Part model, mm, in its own coordinate system. A direction names the side the tool comes from. Coordinates: 2 decimals unless noted, no trailing zeros. Loops run counter-clockwise (first coordinate to the right, second up) from the corner with the lowest first, then second, coordinate; pieces in that order, holes last. Notation, with made-up numbers: (-19, -32.75) -> (30, -32.75) arc R16 cw to (30, -4.75) -> close; hole circle Ø5 at (72, 36). An arc over 180 degrees is marked (long way). Use one line per item in the form item = value. Start each with the question number.
(1) 3-axis set-ups, long thin cutter, end or side, ignore diameter. For faces 4 (the flat face through (35.91, 2, 0.5)), 5 (the flat face through (10.3, -2.658, 0.5)), 6 (the flat face through (10.6, 5.542, 0.5)), 7 (the flat face through (-5.8, -7.658, 0.5)): which of +Z, -Z, +X, -X, +Y, -Y reach the whole face in a straight line?
(2) Band-saw the part on A-A on z = 0.55. Count the separate pieces of the cut face and the enclosed holes in it, then the cut area to 3 significant figures.
(3) Band-saw the part on B-B on y = 2. Give the cut face in (x, z), then the cut area to 3 significant figures.
(4) Mould opens along X. For faces 1 (the flat face through (37.2, 6.542, 0.5)), 2 (the flat face through (40.208, -0.7, 0.5)), 3 (the cylindrical face through (38.46, -0.03, 0.51)) say: +X half, -X half, draft (parallel to the pull), parting line (faces both ways), or undercut.
(5) Band-saw the part on C-C on x = -5. Give the cut face in (y, z), then the cut area to 3 significant figures.
(6) Pin check, flat tips, straight feed: P1, Ø0.5, axis at x = 7.5, z = 0.5, coming from the +Y side; P2, Ø0.5, axis at x = 10, z = 0.5, coming from the -Y side. Stop position of each tip, or through.
(7) Drill centre lines: L1, parallel to X at y = 2, z = 0.85; L2, parallel to X at y = -6, z = 0.4; L3, parallel to X at y = 0, z = 0.2. Where is each one in solid material? Low to high. Write a range as [from, to].
```python
from build123d import *

# Parameters (mm, degrees)
F0_W     = 3
F0_H     = 5
F1_DEPTH = 1
F2_R     = 1.49999
F3_R     = 1.5


# Not quite as in the source:
# - a fillet or chamfer is up to 0.001 mm smaller than in the source, because OpenCascade refuses the exact size


with BuildPart() as f1:
    # F0 (on Top) → F1 (new body)
    with BuildSketch(Plane.XY):
        Polygon((-13.5924067289, 6.5421499412), (-19.5924067289, 6.5421499412), (-19.5924067289, -7.6578500588), (8.3075932711, -7.6578500588), (8.3075932711, -2.6578500588), (12.3075932711, -2.6578500588), (12.3075932711, -7.6578500588), (40.2075932711, -7.6578500588), (40.2075932711, 6.5421499412), (34.2075932711, 6.5421499412), (34.2075932711, 5.5421499412), (-13.5924067289, 5.5421499412), align=None)
        with Locations((-16.332133919, 2.0421499412)):
            Rectangle(F0_W, F0_H, mode=Mode.SUBTRACT)
        with Locations((37.4102636576, 2.0421499412)):
            Rectangle(F0_W, F0_H, mode=Mode.SUBTRACT)
    extrude(amount=F1_DEPTH)

    # F2 (radius 1.5 in the source; OpenCascade refuses exactly that, so slightly less here)
    f2_edges = [f1.edges().sort_by_distance(p)[0] for p in [
        (-17.832134, 4.54215, 0.5),
        (-14.832134, 4.54215, 0.5),
        (-14.832134, -0.45785, 0.5),
        (-17.832134, -0.45785, 0.5),
        (38.910264, 4.54215, 0.5),
        (35.910264, 4.54215, 0.5),
        (35.910264, -0.45785, 0.5),
        (38.910264, -0.45785, 0.5),
    ]]
    fillet(f2_edges, radius=F2_R)

    # F3
    f3_edges = [f1.edges().sort_by_distance(p)[0] for p in [
        (8.307593, -2.65785, 0.5),
        (12.307593, -2.65785, 0.5),
    ]]
    fillet(f3_edges, radius=F3_R)


solid = f1.part
```
A:
q1.face_4 = +Z, -Z
q1.face_5 = +Z, -Z, -Y
q1.face_6 = +Z, -Z, +Y
q1.face_7 = +Z, -Z, +X, -X, -Y
q2.separate_pieces = 1
q2.enclosed_holes = 2
q2.area = 756 mm²
q3.outline = (-19.59, 0) -> (-17.83, 0) -> (-17.83, 1) -> (-19.59, 1) -> close; (-14.83, 0) -> (35.91, 0) -> (35.91, 1) -> (-14.83, 1) -> close; (38.91, 0) -> (40.21, 0) -> (40.21, 1) -> (38.91, 1) -> close
q3.area = 53.8 mm²
q4.face_1 = draft
q4.face_2 = +X half
q4.face_3 = undercut
q5.outline = (-7.66, 0) -> (5.54, 0) -> (5.54, 1) -> (-7.66, 1) -> close
q5.area = 13.2 mm²
q6.P1 = 5.54
q6.P2 = -2.66
q7.L1 = [-19.59, -17.83], [-14.83, 35.91], [38.91, 40.21]
q7.L2 = [-19.59, 8.31], [12.31, 40.21]
q7.L3 = [-19.59, -17.41], [-15.25, 36.33], [38.49, 40.21]
